```python
from build123d import *

# Parameters (mm, degrees)
SKETCH1_W               = 62
SKETCH1_H               = 21.285714286
BOSS_EXTRUDE1_DEPTH     = 12
SKETCH3_R               = 4
BOSS_EXTRUDE2_DEPTH     = 74.5
SKETCH4_OUTSIDE_W       = 51.02
SKETCH4_OUTSIDE_H       = 41.734
SKETCH4_OUTSIDE_R       = 6
CUT_EXTRUDE2_DEPTH      = 137.5
SKETCH5_W               = 4
SKETCH5_H               = 4
CUT_EXTRUDE3_DEPTH      = 7
CUT_EXTRUDE3_DEPTH_BACK = 7
CHAMFER1_SIZE           = 1
CHAMFER1_SIZE2          = 0.577350269


with BuildPart() as part:
    # Sketch1 → Boss-Extrude1 (new body)
    with BuildSketch(Plane(origin=(0, 0, 0), x_dir=(1, 0, 0), z_dir=(0, 1, 0))):
        Rectangle(SKETCH1_W, SKETCH1_H)
    extrude(amount=BOSS_EXTRUDE1_DEPTH)

    # Sketch3 → Boss-Extrude2 (add)
    with BuildSketch(Plane(origin=(31, 0, 0), x_dir=(0, 0, -1), z_dir=(1, 0, 0))):
        with Locations((0, 6)):
            Circle(SKETCH3_R)
    extrude(amount=BOSS_EXTRUDE2_DEPTH)

    # Sketch4 outside → Cut-Extrude2 (cut, through all)
    with BuildSketch(Plane.ZY.offset(31)):
        with Locations((0, 6)):
            Rectangle(SKETCH4_OUTSIDE_W, SKETCH4_OUTSIDE_H)
        with Locations((0, 6)):
            Circle(SKETCH4_OUTSIDE_R, mode=Mode.SUBTRACT)
    extrude(amount=-CUT_EXTRUDE2_DEPTH, mode=Mode.SUBTRACT)

    # Sketch5 → Cut-Extrude3 (cut, two sides)
    with BuildSketch(Plane.XY) as cut_extrude3_sk:
        with BuildLine():
            Line((-19, 8), (-7, 8))
            ThreePointArc((-7, 8), (-5, 6), (-7, 4))
            Line((-7, 4), (-19, 4))
            ThreePointArc((-19, 4), (-21, 6), (-19, 8))
        make_face()
        with Locations((98.5, 6)):
            Rectangle(SKETCH5_W, SKETCH5_H)
    extrude(amount=CUT_EXTRUDE3_DEPTH, mode=Mode.SUBTRACT)
    extrude(cut_extrude3_sk.sketch, amount=-CUT_EXTRUDE3_DEPTH_BACK, mode=Mode.SUBTRACT)

    # Chamfer1
    chamfer1_edges = [part.edges().sort_by_distance(p)[0] for p in [
        (105.5, 6, 4),
    ]]
    chamfer1_side = [part.faces().sort_by_distance(p)[0] for p in [
        (68.25, 6, 4),
    ]]
    chamfer(chamfer1_edges, length=CHAMFER1_SIZE, length2=CHAMFER1_SIZE2, reference=chamfer1_side[0])


solid = part.part
```
Read the model definition and answer for the solid it produces. Units are mm, in the model's axes. A direction names the side the tool comes from. Give positions to 0.01 mm unless a question says otherwise; leave off trailing zeros. Write each loop counter-clockwise with the first axis right and the second up, starting at its lowest first coordinate (ties: lowest second). Pieces come first, ordered by that corner, then holes. Notation, with made-up numbers: (50.25, 34.5) -> (72.25, 34.5) arc R35 ccw to (72.25, 66.5) -> close; hole circle Ø3 at (47, -10.5). An arc over 180 degrees is marked (long way). Answer as a JSON object with one key per item and string values.
1) For a pull along Y with two mould halves and no side action, classify faces 1 (the flat face through (-31, 6, 0)), 2 (the flat face through (96.5, 6, 0)), 3 (the cylindrical face through (-0.434, 0.677, 2.769)) as pulls with the +Y half, pulls with the -Y half, needs draft (parallel to the pull), parting line crosses it, or undercut.
Findings below:
{"face 1": "needs draft", "face 2": "undercut", "face 3": "parting line crosses it"}
2) Section B-B on z = 0 is taken. Write down the section's boundary in (x, y).
Findings below:
{"outline": "(-31, 0) -> (31, 0) -> (31, 2) -> (104.5, 2) -> (105.5, 2.58) -> (105.5, 9.42) -> (104.5, 10) -> (31, 10) -> (31, 12) -> (-31, 12) -> close; hole (-19, 4) -> (-7, 4) arc R2 ccw to (-7, 8) -> (-19, 8) arc R2 ccw to start; hole (96.5, 4) -> (100.5, 4) -> (100.5, 8) -> (96.5, 8) -> close"}
3) Section A-A on y = 6 is taken. Write down the section's boundary in (x, z), then the cut area to 3 significant figures.
Findings below:
{"outline": "(-31, -6) -> (-21, -6) -> (-21, 6) -> (-31, 6) -> close; (-5, -6) -> (31, -6) -> (31, -4) -> (96.5, -4) -> (96.5, 4) -> (31, 4) -> (31, 6) -> (-5, 6) -> close; (100.5, -4) -> (104.5, -4) -> (105.5, -3.42) -> (105.5, 3.42) -> (104.5, 4) -> (100.5, 4) -> close", "area": "1,120 mm^2"}
4) Section C-C on x = 4 is taken. Write down the section's boundary in (y, z), then the cut area to 3 significant figures.
Findings below:
{"outline": "circle Ø12 at (6, 0)", "area": "113 mm^2"}
5) Section D-D on x = 50.5 is taken. Write down the section's boundary in (y, z), then the cut area to 3 significant figures.
Findings below:
{"outline": "circle Ø8 at (6, 0)", "area": "50.3 mm^2"}
6) A tool of negligible diameter and unlimited length cuts with its end or side. For faces 4 (the cylindrical face through (67, 6, 4)), 5 (the flat face through (-13, 8, 0)), 6 (the flat face through (105.5, 6, 0)), from which of +Z, -Z, +X, -X, +Y, -Y can it reach the whole face along a straight path? Write none if from no direction.
Findings below:
{"face 4": "+X", "face 5": "+Z, -Z", "face 6": "+Z, -Z, +X, +Y, -Y"}
7) Straight lines are drawn through the part: probe 1 along X at (y, z) = (6, -3); probe 2 along X at (y, z) = (7.5, 0); probe 3 along X at (y, z) = (7.75, -4.25). For each, find the intervals that lie inside material, in ascending order. Write a range as from..to.
Findings below:
{"probe 1": "x = -31..-21, -5..96.5, 100.5..105.5", "probe 2": "x = -31..-20.32, -5.68..96.5, 100.5..105.5", "probe 3": "x = -31..-19.97, -6.03..31"}
8) Flat-ended cylindrical pins translate along their axes: pin 1 Ø2 at (x, z) = (99, -1) entering from -Y; pin 2 Ø1.5 at (x, y) = (19.5, 8) entering from +Z; pin 3 Ø4 at (x, z) = (38.5, -2.5) entering from +Y. Find the tip coordinate at first contact, or state that the pin passes through.
Findings below:
{"pin 1": "stops at y = 2", "pin 2": "stops at z = 5.87", "pin 3": "stops at y = 9.97"}
